Design review of the part built by this model. Coordinates are the model's own, in mm. A direction names the side the tool comes from. Coordinates: 2 decimals unless noted, no trailing zeros. Loops run counter-clockwise (first coordinate to the right, second up) from the corner with the lowest first, then second, coordinate; pieces in that order, holes last. Notation, with made-up numbers: (74.25, 65) -> (85.25, 65) arc R31 cw to (85.25, 103) -> close; hole circle Ø2 at (63.5, 66). An arc over 180 degrees is marked (long way). Use one line per item in the form item = value. Start each with the question number.
1. Wall thickness on line 1 (Y direction, x = 0, z = 1.7); line 2 (X direction, y = 30, z = 0.9) (3 decimals); line 3 (Y direction, x = -21.4, z = 2.1): over which ranges is each line inside the solid? List them lowest first. Write a range as from..to.
2. Consider section C-C (y = 40). State the section outline as (x, z) points (3 decimals).
3. Machinability: for faces 1 (the face through (20, 27.5, 2)), 2 (the face through (0, 10, 2)), which of the approach directions +Z, -Z, +X, -X, +Y, -Y give a long, thin tool a straight path to every point of the face, cutting with its end or side? Answer none if there is none.
4. Consider section A-A (x = 0). State the section outline as (y, z) points (3 decimals), then the cut area to 3 significant figures.
5. The part is to be moulded in two halves that separate along X. For faces 3 (the face through (-26.485, 28.298, 1.61)), 4 (the face through (-21.93, 40.27, 1.57)), 5 (the face through (33, 19, 2)), say which applies: released by +X, released by -X, zero draft, split by the parting line, or undercut.
6. For pin 1 (1 mm diameter, centred on y = 40.5, z = 2, fed in from -X) (3 decimals); pin 2 (1.5 mm diameter, centred on x = -19.5, y = 36, fed in from +Z); pin 3 (1 mm diameter, centred on y = 37, z = 1.5, fed in from +X), all flat-tipped, find the tip position at first contact; note any pin that passes through.
7. Consider section D-D (y = 17.5). State the section outline as (x, z) points (3 decimals), then the cut area to 3 significant figures.
8. Consider section B-B (z = 1.8). State the section outline as (x, y) points, then the cut area to 3 significant figures.
from build123d import *

# Parameters (mm, degrees)
SKETCH1_W           = 19.6
SKETCH1_H           = 47
SKETCH1_R           = 2.5527
SKETCH1_R_2         = 7
BOSS_EXTRUDE1_DEPTH = 3.175
SKETCH2_W           = 23.2
SKETCH2_H           = 15
SKETCH2_R           = 2.5527
BOSS_EXTRUDE2_DEPTH = 3.175
BOSS_EXTRUDE3_DEPTH = 3.175
FILLET1_R           = 2.5
FILLET2_R           = 1.5
FILLET3_R           = 2.5


with BuildPart() as part:
    # Sketch1 → Boss-Extrude1 (new body)
    with BuildSketch(Plane.XY):
        with Locations((0, 33.5)):
            Rectangle(SKETCH1_W, SKETCH1_H)
        with Locations((0, 17.5)):
            Circle(SKETCH1_R, mode=Mode.SUBTRACT)
        with Locations((0, 40)):
            Circle(SKETCH1_R_2, mode=Mode.SUBTRACT)
    extrude(amount=BOSS_EXTRUDE1_DEPTH)

    # Sketch2 → Boss-Extrude2 (add)
    # profile 1 of 2: a face of its own
    with BuildSketch(Plane.XY.offset(3.175)):
        with Locations((21.4, 17.5)):
            Rectangle(SKETCH2_W, SKETCH2_H)
        with Locations((21.4, 17.5)):
            Circle(SKETCH2_R, mode=Mode.SUBTRACT)
    # profile 2 of 2: a face of its own
    with BuildSketch(Plane.XY.offset(3.175)):
        with Locations((-21.4, 17.5)):
            Rectangle(SKETCH2_W, SKETCH2_H)
        with Locations((-21.4, 17.5)):
            Circle(SKETCH2_R, mode=Mode.SUBTRACT)
    extrude(amount=-BOSS_EXTRUDE2_DEPTH)

    # Sketch3 → Boss-Extrude3 (add)
    # profile 1 of 2: a face of its own
    with BuildSketch(Plane(origin=(0, 0, 0), x_dir=(-1, 0, 0), z_dir=(0, 0, -1))):
        Polygon((33, 25), (9.8, 57), (9.8, 25), align=None)
        Polygon((28.099595168, 27.5), (12.3, 49.29254506), (12.3, 27.5), align=None, mode=Mode.SUBTRACT)
    # profile 2 of 2: a face of its own
    with BuildSketch(Plane(origin=(0, 0, 0), x_dir=(-1, 0, 0), z_dir=(0, 0, -1))):
        Polygon((-9.8, 57), (-33, 25), (-9.8, 25), align=None)
        Polygon((-12.3, 49.29254506), (-28.099595168, 27.5), (-12.3, 27.5), align=None, mode=Mode.SUBTRACT)
    extrude(amount=-BOSS_EXTRUDE3_DEPTH)

    # Fillet1
    fillet1_edges = [part.edges().sort_by_distance(p)[0] for p in [
        (-12.3, 27.5, 1.5875),
        (12.3, 27.5, 1.5875),
    ]]
    fillet(fillet1_edges, radius=FILLET1_R)

    # Fillet2
    fillet2_edges = [part.edges().sort_by_distance(p)[0] for p in [
        (-12.3, 49.29254506, 1.5875),
        (-28.099595168, 27.5, 1.5875),
        (28.099595168, 27.5, 1.5875),
        (12.3, 49.29254506, 1.5875),
    ]]
    fillet(fillet2_edges, radius=FILLET2_R)

    # Fillet3
    fillet3_edges = [part.edges().sort_by_distance(p)[0] for p in [
        (-9.8, 57, 1.5875),
        (9.8, 57, 1.5875),
        (33, 10, 1.5875),
        (-33, 10, 1.5875),
    ]]
    fillet(fillet3_edges, radius=FILLET3_R)


solid = part.part
Geometry check:
q1.line_1 = 10..14.95, 20.05..33, 47..57
q1.line_2 = -29.375..-26.287, -12.3..12.3, 26.287..29.375
q1.line_3 = 10..14.95, 20.05..27.5, 36.74..41
q2.outline = (-22.125, 0) -> (-19.037, 0) -> (-19.037, 3.175) -> (-22.125, 3.175) -> close; (-12.3, 0) -> (-7, 0) -> (-7, 3.175) -> (-12.3, 3.175) -> close; (7, 0) -> (12.3, 0) -> (12.3, 3.175) -> (7, 3.175) -> close; (19.037, 0) -> (22.125, 0) -> (22.125, 3.175) -> (19.037, 3.175) -> close
q3.face_1 = +Z, -Z
q3.face_2 = +Z, -Z, +X, -X, -Y
q4.outline = (10, 0) -> (14.947, 0) -> (14.947, 3.175) -> (10, 3.175) -> close; (20.053, 0) -> (33, 0) -> (33, 3.175) -> (20.053, 3.175) -> close; (47, 0) -> (57, 0) -> (57, 3.175) -> (47, 3.175) -> close
q4.area = 88.6 mm²
q5.face_3 = undercut
q5.face_4 = released by -X
q5.face_5 = released by +X
q6.pin_1 = -22.125
q6.pin_2 = through
q6.pin_3 = 24.66
q7.outline = (-33, 0) -> (-23.953, 0) -> (-23.953, 3.175) -> (-33, 3.175) -> close; (-18.847, 0) -> (-2.553, 0) -> (-2.553, 3.175) -> (-18.847, 3.175) -> close; (2.553, 0) -> (18.847, 0) -> (18.847, 3.175) -> (2.553, 3.175) -> close; (23.953, 0) -> (33, 0) -> (33, 3.175) -> (23.953, 3.175) -> close
q7.area = 161 mm²
q8.outline = (-33, 12.5) arc R2.5 ccw to (-30.5, 10) -> (30.5, 10) arc R2.5 ccw to (33, 12.5) -> (33, 25) -> (10.55, 55.97) arc R2.5 ccw to (8.52, 57) -> (-8.52, 57) arc R2.5 ccw to (-10.55, 55.97) -> (-33, 25) -> close; hole (-26.37, 29.88) arc R1.5 ccw to (-25.16, 27.5) -> (-14.8, 27.5) arc R2.5 ccw to (-12.3, 30) -> (-12.3, 44.67) arc R1.5 ccw to (-15.01, 45.55) -> close; hole circle Ø5.11 at (-21.4, 17.5); hole circle Ø14 at (0, 40); hole circle Ø5.11 at (0, 17.5); hole (12.3, 30) arc R2.5 ccw to (14.8, 27.5) -> (25.16, 27.5) arc R1.5 ccw to (26.37, 29.88) -> (15.01, 45.55) arc R1.5 ccw to (12.3, 44.67) -> close; hole circle Ø5.11 at (21.4, 17.5)
q8.area = 1,810 mm²
